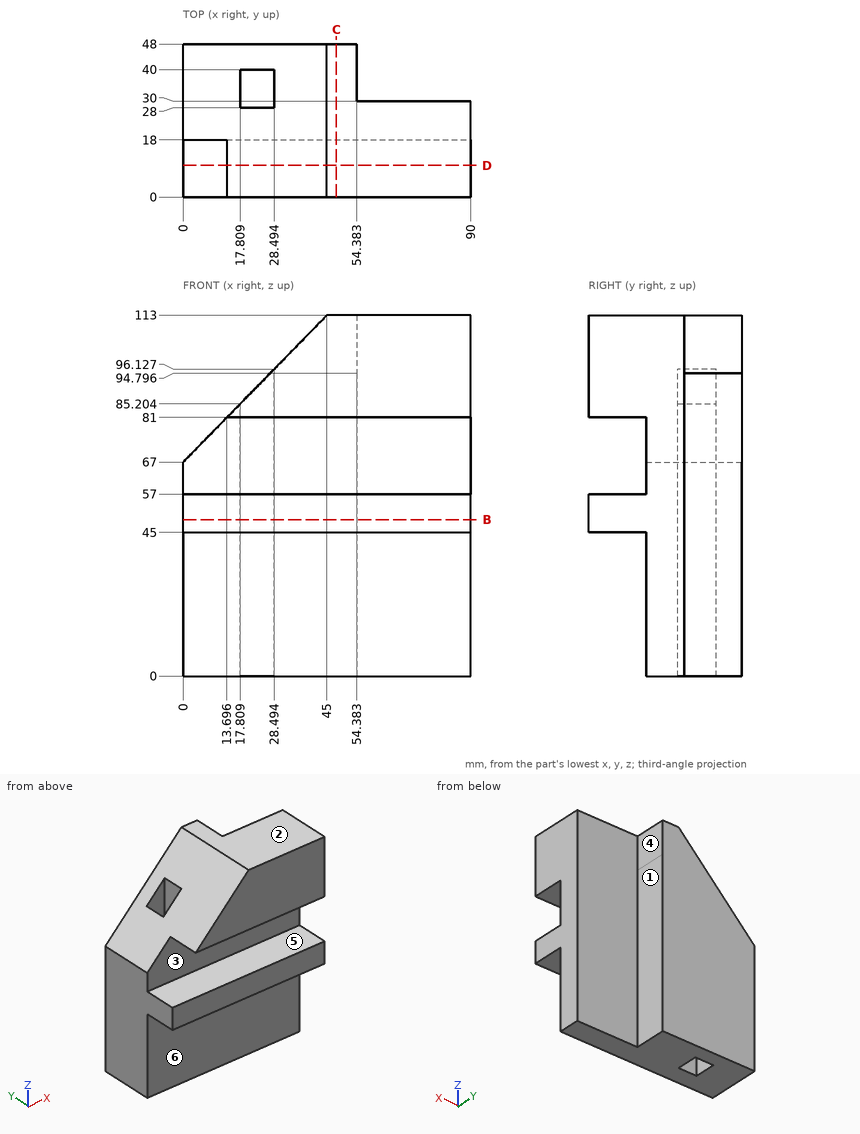
Study the drawing (mm; zero at the part's minimum x, y, z) and answer. A direction names the side the tool comes from. Coordinates: 2 decimals unless noted, no trailing zeros. Order: outer loops, then holes, each group sorted by start corner. A loop starts at its lowest first (then second) coordinate and runs counter-clockwise, first axis right, second up. Notation, with made-up numbers: M 43.25,27 L 79.25,27 A20 ccw 79.25,57 Z; hole C -6,11 d10. An arc over 180 degrees is marked long. Use CSV: the item, a comma, the result in double quotes.
Q1. Section C-C (x = 48) is taken. Determine the outline of the cut face in (y, z), then the cut area to 3 significant figures.
Here are the results:
outline,"M 0,45 L 18,45 L 18,0 L 48,0 L 48,113 L 0,113 L 0,81 L 18,81 L 18,57 L 0,57 Z"
area,"4,180 mm2"
Q2. Determine the mould class of the marked faces 1, 2 and 3 for opening direction Z: pulls with the +Z half, pulls with the -Z half, needs draft (parallel to the pull), parting line crosses it, or undercut.
Here are the results:
face 1,"needs draft"
face 2,"pulls with the +Z half"
face 3,"undercut"
Q3. Section D-D (y = 10) is taken. Determine the outline of the cut face in (x, z) (1 decimal), then the cut area to 3 significant figures.
Here are the results:
outline,"M 0,45 L 90,45 L 90,57 L 0,57 Z; M 13.7,81 L 90,81 L 90,113 L 45,113 Z"
area,"3,020 mm2"
Q4. Given pin 1 Ø8 at (y, z) = (8, 90.5) entering from -X (1 decimal); pin 2 Ø5.5 at (y, z) = (38.5, 104) entering from +X; pin 3 Ø6 at (x, z) = (26, 28) entering from -Y, each flat-ended and moving along its own axis, determine where each tip first touches the part or whether it passes through.
Here are the results:
pin 1,"x = 19.1"
pin 2,"x = 54.38"
pin 3,"y = 18"
Q5. Straight lines are drawn through the part: L1, parallel to Z at x = 48, y = 9; L2, parallel to X at y = 32, z = 60.5; L3, parallel to Y at x = 27, z = 64.5. For each, find the intervals that lie inside material, in ascending order.
Here are the results:
L1,"45 to 57, 81 to 113"
L2,"0 to 17.81, 28.49 to 54.38"
L3,"18 to 28, 40 to 48"
Q6. Section B-B (z = 49) is taken. Determine the outline of the cut face in (x, y), then the cut area to 3 significant figures.
Here are the results:
outline,"M 0,0 L 90,0 L 90,30 L 54.38,30 L 54.38,48 L 0,48 Z; hole M 17.81,28 L 28.49,28 L 28.49,40 L 17.81,40 Z"
area,"3,550 mm2"
Q7. A tool of negligible diameter and unlimited length cuts with its end or side. For the marked faces 4, 5 and 6, from which of +Z, -Z, +X, -X, +Y, -Y can it reach the whole face along a straight path? Write none if from no direction.
Here are the results:
face 4,"+Z, -Z, +X, +Y"
face 5,"+X, -X, -Y"
face 6,"-Z, +X, -X, -Y"
